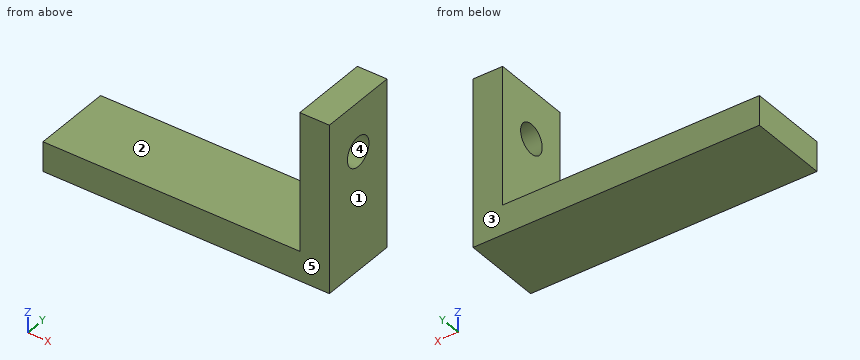
```python
from build123d import *

# Parameters (mm, degrees)
F1_DEPTH = 8
F2_R     = 1.5
F3_DEPTH = 25


with BuildPart() as f1:
    # F0 (on Front) → F1 (new body)
    with BuildSketch(Plane.XZ):
        Polygon((1.5, 8.5), (-1.5, 8.5), (-1.5, -5.5), (-27.5, -5.5), (-27.5, -8.5), (-1.5, -8.5), (1.5, -8.5), align=None)
    extrude(amount=F1_DEPTH)

    # F2 (on face) → F3 (cut)
    with BuildSketch(Plane.YZ.offset(1.5)):
        with Locations((-4, 3.5)):
            Circle(F2_R)
    extrude(amount=-F3_DEPTH, mode=Mode.SUBTRACT)


solid = f1.part
```
Check sheet for the modelled part. Datum: model origin and axes. Units: mm. Face numbers are marked on the shaded views. A direction names the side the tool comes from. Give positions to 0.01 mm unless a question says otherwise; leave off trailing zeros. Order: outer loops, then holes, each group sorted by start corner. A loop starts at its lowest first (then second) coordinate and runs counter-clockwise, first axis right, second up. Notation, with made-up numbers: (-39.75, -28.75) -> (-18.75, -28.75) arc R13 cw to (-18.75, -9.75) -> close; hole circle Ø1 at (-22, 60). An arc over 180 degrees is marked (long way). Use CSV: the item, a comma, the result in double quotes. Start each with the question number.
1) Sectioned sample at C-C, the plane y = -1. Record the boundary of the cut face in (x, z).
2) Set-up check for the marked faces 1 and 2: record each of +Z, -Z, +X, -X, +Y, -Y from which the full face is reachable in a straight line by a thin tool's end or side.
3) Sectioned sample at A-A, the plane y = -4. Record the boundary of the cut face in (x, z).
4) Go/stop test with flat-tipped pins: P1, Ø4, axis at x = -18.5, y = -5, coming from the +Z side; P2, Ø1, axis at y = -1.5, z = 3, coming from the -X side. Record where each tip stops, or that it passes through.
5) Mould release check, pull along Y, two halves, no side actions. Record for the marked faces 3, 4 and 5: released by +Y, released by -Y, zero draft, split by the parting line, or undercut.
6) Sectioned sample at B-B, the plane z = 3.5. Record the boundary of the cut face in (x, y).
7) Sectioned sample at D-D, the plane x = -9.5. Record the boundary of the cut face in (y, z), plus the area to 3 significant figures.
8) Material ranges on line 1 (Z direction, x = 0.15, y = -4); line 2 (Z direction, x = -24.5, y = -3); line 3 (X direction, y = -3.25, z = -4.5), recorded low to high. Write a range as from..to.
Recorded:
1,outline,"(-27.5, -8.5) -> (1.5, -8.5) -> (1.5, 8.5) -> (-1.5, 8.5) -> (-1.5, -5.5) -> (-27.5, -5.5) -> close"
2,face 1,"+Z, -Z, +X, +Y, -Y"
2,face 2,"+Z, -X, +Y, -Y"
3,outline,"(-27.5, -8.5) -> (1.5, -8.5) -> (1.5, 2) -> (-1.5, 2) -> (-1.5, -5.5) -> (-27.5, -5.5) -> close; (-1.5, 5) -> (1.5, 5) -> (1.5, 8.5) -> (-1.5, 8.5) -> close"
4,P1,"z = -5.5"
4,P2,"x = -1.5"
5,face 3,"released by +Y"
5,face 4,"undercut"
5,face 5,"released by -Y"
6,outline,"(-1.5, -8) -> (1.5, -8) -> (1.5, -5.5) -> (-1.5, -5.5) -> close; (-1.5, -2.5) -> (1.5, -2.5) -> (1.5, 0) -> (-1.5, 0) -> close"
7,outline,"(-8, -8.5) -> (0, -8.5) -> (0, -5.5) -> (-8, -5.5) -> close"
7,area,"24.0 mm2"
8,line 1,"-8.5..2, 5..8.5"
8,line 2,"-8.5..-5.5"
8,line 3,"-1.5..1.5"
